Input: part model. Units: mm. Frame: model coordinates. A direction names the side the tool comes from. Coordinates: 2 decimals unless noted, no trailing zeros. Order: outer loops, then holes, each group sorted by start corner. A loop starts at its lowest first (then second) coordinate and runs counter-clockwise, first axis right, second up. Notation, with made-up numbers: (15, -11.5) -> (44, -11.5) arc R17 ccw to (44, -1.5) -> close; hole circle Ø3 at (87, -5). An arc over 180 degrees is marked (long way). One line per question, with ' | ' between items.
```python
from build123d import *

# Parameters (mm, degrees)
SKETCH_1_W          = 10
SKETCH_1_H          = 10
SKETCH_1_W_2        = 8
SKETCH_1_H_2        = 8
EXTRUDE_1_DEPTH     = 120
SKETCH_3_R          = 1.5
CUT_EXTRUDE_1_DEPTH = 121.519707932
SKETCH_4_R          = 1.5
CUT_EXTRUDE_2_DEPTH = 121.519707932


with BuildPart() as part:
    # ｽｹｯﾁ1 → 押し出し-薄板1 (new body)
    with BuildSketch(Plane(origin=(0, 0, 0), x_dir=(0, 0, -1), z_dir=(1, 0, 0))):
        Rectangle(SKETCH_1_W, SKETCH_1_H)
        Rectangle(SKETCH_1_W_2, SKETCH_1_H_2, mode=Mode.SUBTRACT)
    extrude(amount=EXTRUDE_1_DEPTH)

    # ｽｹｯﾁ3 → ｶｯﾄ - 押し出し1 (cut, through all)
    with BuildSketch(Plane.XY.offset(5)):
        with Locations((115, 0)):
            Circle(SKETCH_3_R)
        with Locations((10, 0)):
            Circle(SKETCH_3_R)
        with Locations((20.25, 0)):
            Circle(SKETCH_3_R)
        with Locations((5, 0)):
            Circle(SKETCH_3_R)
    extrude(amount=-CUT_EXTRUDE_1_DEPTH, mode=Mode.SUBTRACT)

    # ｽｹｯﾁ4 → ｶｯﾄ - 押し出し2 (cut, through all)
    with BuildSketch(Plane(origin=(0, 5, 0), x_dir=(1, 0, 0), z_dir=(0, 1, 0))):
        with Locations(Location((5, 0, 0), (0, 0, 270))):
            Circle(SKETCH_4_R)
        with Locations(Location((45, 0, 0), (0, 0, 270))):
            Circle(SKETCH_4_R)
        with Locations(Location((75, 0, 0), (0, 0, 270))):
            Circle(SKETCH_4_R)
    extrude(amount=-CUT_EXTRUDE_2_DEPTH, mode=Mode.SUBTRACT)


solid = part.part
```
1. Cut plane B-B, the plane z = 0. State how many separate pieces and enclosed holes the cut face has, and give its area (3 significant figures).
Recorded:
separate pieces: 8 | enclosed holes: 0 | area: 222 mm^2
2. Cut plane C-C, the plane y = 3. Return loops of the section in (x, z), and give its area (3 significant figures).
Recorded:
outline: (0, -5) -> (120, -5) -> (120, -4) -> (0, -4) -> close; (0, 4) -> (120, 4) -> (120, 5) -> (0, 5) -> close | area: 240 mm^2
3. Cut plane D-D, the plane x = 71. Return loops of the section in (y, z), and give its area (3 significant figures).
Recorded:
outline: (-5, -5) -> (5, -5) -> (5, 5) -> (-5, 5) -> close; hole (-4, -4) -> (4, -4) -> (4, 4) -> (-4, 4) -> close | area: 36.0 mm^2
4. Cut plane A-A, the plane x = 20.25. Return loops of the section in (y, z).
Recorded:
outline: (-5, -5) -> (-1.5, -5) -> (-1.5, -4) -> (-4, -4) -> (-4, 4) -> (-1.5, 4) -> (-1.5, 5) -> (-5, 5) -> close; (1.5, -5) -> (5, -5) -> (5, 5) -> (1.5, 5) -> (1.5, 4) -> (4, 4) -> (4, -4) -> (1.5, -4) -> close
5. Ray query, line 1 (Z direction, x = 37.5, y = 0.5); line 2 (Y direction, x = 5, z = 4.7). Return the intervals inside material, ascending. Write a range as [from, to].
Recorded:
line 1: z = [-5, -4], [4, 5] | line 2: y = [-5, -1.5], [1.5, 5]
6. Mould query, pull axis Y, two halves, no side actions, for faces 3 (the face through (59, -5, 0)), 4 (the face through (0, 0.1, 4.5)), 5 (the face through (113.5, 0.07, -4.49)). Classes: released by +Y, released by -Y, zero draft, split by the parting line, or undercut.
Recorded:
face 3: released by -Y | face 4: zero draft | face 5: undercut
7. Access query for faces 1 (the face through (59, 0, -4)), 2 (the face through (6.386, -0.575, -4.493)). Directions: +Z, -Z, +X, -X, +Y, -Y. A direction counts if a zero-diameter tool reaches every point of the face in a straight line with its end or side. Return the directions, or none.
Recorded:
face 1: +X, -X | face 2: +Z, -Z
